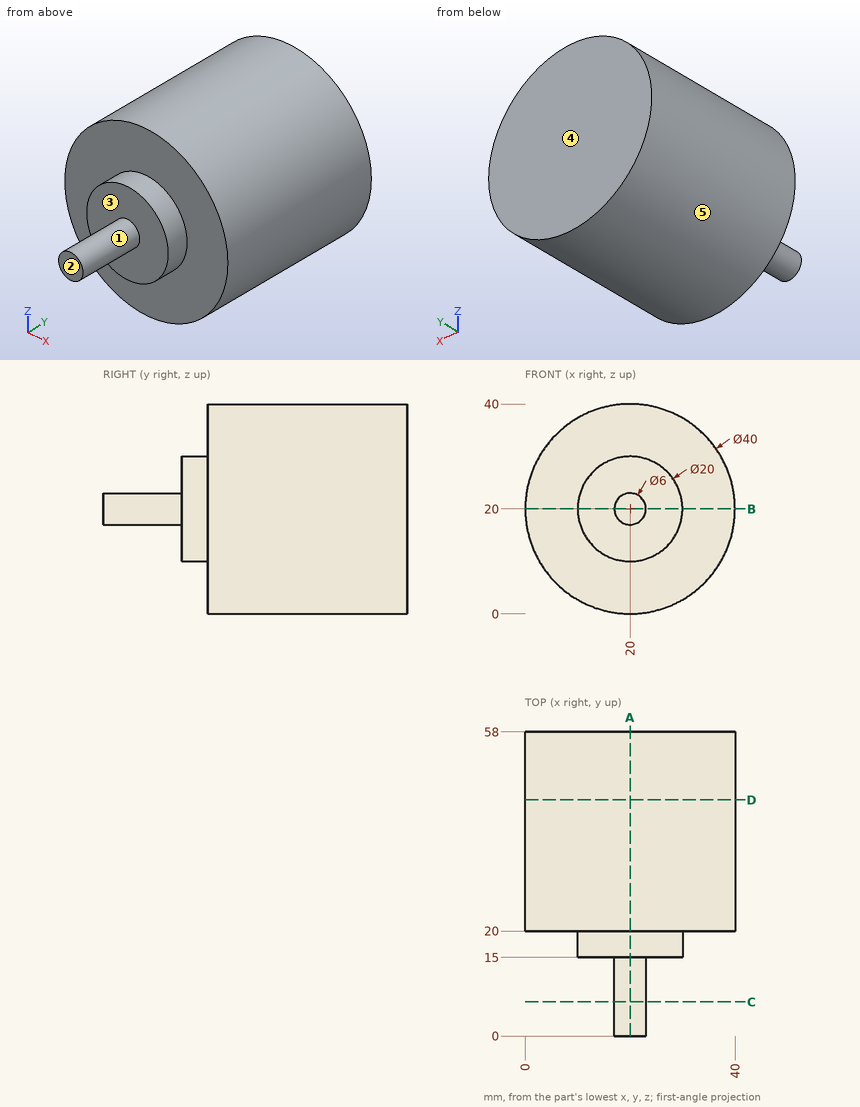
Part print with two shaded views. Sizes in mm from the minimum x, y, z corner. A direction names the side the tool comes from. Round coordinates to 2 decimals unless told otherwise and drop trailing zeros. Write each loop counter-clockwise with the first axis right and the second up, starting at its lowest first coordinate (ties: lowest second). Pieces come first, ordered by that corner, then holes. Notation, with made-up numbers: (24.5, 79.25) - (49.5, 79.25) arc R27 ccw to (49.5, 107.25) - close; hole circle Ø9 at (3, -17). An arc over 180 degrees is marked (long way). Use CSV: the item, a comma, the result in double quotes.
Item 1: Slice it at A-A, the plane x = 20. Write the cut outline in (y, z), then the cut area to 3 significant figures.
Results list:
outline,"(0, 17) - (15, 17) - (15, 10) - (20, 10) - (20, 0) - (58, 0) - (58, 40) - (20, 40) - (20, 30) - (15, 30) - (15, 23) - (0, 23) - close"
area,"1,710 mm²"
Item 2: Slice it at C-C, the plane y = 6.5. Write the cut outline in (x, z).
Results list:
outline,"circle Ø6 at (20, 20)"
Item 3: Slice it at D-D, the plane y = 45. Write the cut outline in (x, z), then the cut area to 3 significant figures.
Results list:
outline,"circle Ø40 at (20, 20)"
area,"1,260 mm²"
Item 4: Pull direction Y, two halves, no side cores. Call the marked faces 3, 4 and 5: pulls with the +Y half, pulls with the -Y half, needs draft (parallel to the pull), parting line crosses it, or undercut.
Results list:
face 3,"pulls with the -Y half"
face 4,"pulls with the +Y half"
face 5,"needs draft"
Item 5: Wall check: L1, parallel to Y at x = 30, z = 25; L2, parallel to Y at x = 17, z = 19; L3, parallel to Z at x = 37.5, y = 24. Give the ranges that are in metal, low to high.
Results list:
L1,"y = 20 to 58"
L2,"y = 15 to 58"
L3,"z = 10.32 to 29.68"
Item 6: Tool access for the marked faces 1 and 2: list every direction of +Z, -Z, +X, -X, +Y, -Y with a clear straight run to the whole face (end or side of a thin tool).
Results list:
face 1,"-Y"
face 2,"+Z, -Z, +X, -X, -Y"
Item 7: Slice it at B-B, the plane z = 20. Write the cut outline in (x, y), then the cut area to 3 significant figures.
Results list:
outline,"(0, 20) - (10, 20) - (10, 15) - (17, 15) - (17, 0) - (23, 0) - (23, 15) - (30, 15) - (30, 20) - (40, 20) - (40, 58) - (0, 58) - close"
area,"1,710 mm²"
Item 8: Flat gauge pins, fed straight in: P1, Ø1.5, axis at x = 34.5, y = 52, coming from the +Z side; P2, Ø10, axis at x = 32.5, y = 47, coming from the -Z side; P3, Ø4, axis at x = 27, y = 43, coming from the +Z side. Where does each tip first touch, or does it go through?
Results list:
P1,"stops at z = 34.52"
P2,"stops at z = 1.46"
P3,"stops at z = 39.36"
